Autodesk Inventor part; units mm, degrees
ref_plane "YZ Plane" through (0, 0, 0) normal (1, 0, 0) x (0, 1, 0)
ref_plane "XZ Plane" through (0, 0, 0) normal (0, 1, 0) x (-1, 0, 0)
ref_plane "XY Plane" through (0, 0, 0) normal (0, 0, 1) x (1, 0, 0)
sketch "Sketch1" plane through (0, 0, 0) normal (1, 0, 0) x (0, 1, 0)
  line L0 (0, 0) -> (8.75, 0) construction
  line L1 (8.75, 0) -> (8.75, -2)
  line L2 (8.75, -2) -> (8.9374, -2)
  line L3 (8.9374, -2) -> (8.9374, -4.5)
  line L4 (8.9374, -4.5) -> (8.75, -4.5)
  line L5 (8.75, -4.5) -> (8.75, -5.5)
  line L6 (8.75, -5.5) -> (13, -5.5)
  line L7 (13, -5.5) -> (13, -10.5)
  line L8 (13, -10.5) -> (16, -10.5)
  line L9 (16, -10.5) -> (16, 0)
  line L10 (16, 0) -> (8.75, 0)
  line L11 (0, 0) -> (0, -14.519)
  dimension "d0" = 8.75
  dimension "d1" = 2
  dimension "d2" = 2.5
  dimension "d3" = 1
  dimension "d4" = 5
  dimension "d5" = 13
  dimension "d8" = 16
revolve "Revolution1" add sketch "Sketch1" angle 200 about axis through (0, 0, 0) along (0, 0, -1)
properties part number "00_Adapter_M8_Fluorescentfilter_Cellphone"
Work out the finished part from the listing and answer in its coordinate system (mm). A direction names the side the tool comes from. Give positions to 0.01 mm unless a question says otherwise; leave off trailing zeros. Loops run counter-clockwise (first coordinate to the right, second up) from the corner with the lowest first, then second, coordinate; pieces in that order, holes last. Notation, with made-up numbers: (65, 88.5) -> (92, 88.5) arc R25 ccw to (92, 100.5) -> close; hole circle Ø9 at (86, 77.25). An arc over 180 degrees is marked (long way). Put each result on its own line as item: value. Start each with the question number.
Item 1: Each of these flat-tipped pins is pushed along its axis until it touches: P1, Ø1.5, axis at y = -4.5, z = -7, coming from the -X side; P2, Ø2, axis at x = 5.5, z = -6.5, coming from the +Y side. Where does it stop, or does it pass through?
Item 2: Which of the six approach directions +Z, -Z, +X, -X, +Y, -Y give full straight-line access (tool end or side, diameter ignored) to faces 5 (the face through (0, 13, -4)), 6 (the face through (12.854, -1.944, -8.035)), 7 (the face through (8.65, -1.31, -1.01))?
Item 3: The part is cut by section D-D (z = -9.25). Give the vertices of the cut face in (x, y).
Item 4: The mould has two halves that part along Z. Classify faces 1 (the face through (13.3, -0.1, -10.5)), 2 (the face through (8.837, -1.336, -3.268)), 3 (the face through (10, 0, 0)), 4 (the face through (15.684, -3.163, -5.176)): released by +Z, released by -Z, zero draft, split by the parting line, or undercut.
Item 5: The part is cut by section C-C (y = 8). Give the vertices of the cut face in (x, z).
Item 6: Find the intervals of material crossed by L1, parallel to Z at x = 5, y = 11; L2, parallel to X at y = 0, z = -5.05; L3, parallel to Y at x = 10.5, z = -6.75, in increasing order. Write a range as [from, to].
Item 7: The part is cut by section A-A (y = 0). Give the vertices of the cut face in (x, z), then the cut area to 3 significant figures.
Item 8: The part is cut by section B-B (x = 1). Give the vertices of the cut face in (y, z).
Answers below:
1. P1: x = 11.89
1. P2: y = 15.35
2. face 5: +Z, -Z, -X, +Y
2. face 6: -Z
2. face 7: +Z, -Z
3. outline: (-5.47, -15.04) arc R16 ccw (long way) to (0, 16) -> (0, 13) arc R13 cw (long way) to (-4.45, -12.22) -> close
4. face 1: released by -Z
4. face 2: undercut
4. face 3: released by +Z
4. face 4: zero draft
5. outline: (3.54, -5.5) -> (10.25, -5.5) -> (10.25, -10.5) -> (13.86, -10.5) -> (13.86, 0) -> (3.54, 0) -> (3.54, -2) -> (3.98, -2) -> (3.98, -4.5) -> (3.54, -4.5) -> close
6. L1: [-5.5, 0]
6. L2: [8.75, 16]
6. L3: [-12.07, -7.66], [7.66, 12.07]
7. outline: (8.75, -5.5) -> (13, -5.5) -> (13, -10.5) -> (16, -10.5) -> (16, 0) -> (8.75, 0) -> (8.75, -2) -> (8.94, -2) -> (8.94, -4.5) -> (8.75, -4.5) -> close
7. area: 54.4 mm2
8. outline: (-15.97, -10.5) -> (-12.96, -10.5) -> (-12.96, -5.5) -> (-8.69, -5.5) -> (-8.69, -4.5) -> (-8.88, -4.5) -> (-8.88, -2) -> (-8.69, -2) -> (-8.69, 0) -> (-15.97, 0) -> close; (8.69, -5.5) -> (12.96, -5.5) -> (12.96, -10.5) -> (15.97, -10.5) -> (15.97, 0) -> (8.69, 0) -> (8.69, -2) -> (8.88, -2) -> (8.88, -4.5) -> (8.69, -4.5) -> close
